Part model, mm, in its own coordinate system. Give positions to 0.01 mm unless a question says otherwise; leave off trailing zeros. Loops run counter-clockwise (first coordinate to the right, second up) from the corner with the lowest first, then second, coordinate; pieces in that order, holes last. Notation, with made-up numbers: (9, 72.5) -> (47, 72.5) arc R11 ccw to (47, 89.5) -> close; hole circle Ø9 at (27.25, 8.25). An arc over 180 degrees is marked (long way). One line per question, with ' | ' between items.
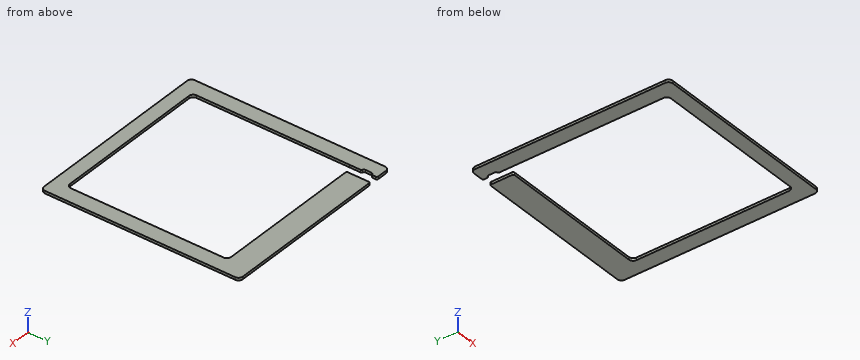
```python
from build123d import *

# Parameters (mm, degrees)
SKETCH1_W           = 323.85
SKETCH1_H           = 336.55
BOSS_EXTRUDE1_DEPTH = 4.3434
SKETCH2_W           = 271.78
SKETCH2_H           = 273.05
CUT_EXTRUDE1_DEPTH  = 5.3434
FILLET1_R           = 7.14375
CUT_EXTRUDE2_DEPTH  = 5.3434
SKETCH4_W           = 14.979655554
SKETCH4_H           = 46.925096095
CUT_EXTRUDE3_DEPTH  = 5.3434
FILLET2_R           = 2.54


with BuildPart() as part:
    # Sketch1 → Boss-Extrude1 (new body)
    with BuildSketch(Plane.XY):
        Rectangle(SKETCH1_W, SKETCH1_H)
    extrude(amount=BOSS_EXTRUDE1_DEPTH)

    # Sketch2 → Cut-Extrude1 (cut, through all)
    with BuildSketch(Plane.XY.offset(4.3434)):
        with Locations((0, -8.382)):
            Rectangle(SKETCH2_W, SKETCH2_H)
    extrude(amount=-CUT_EXTRUDE1_DEPTH, mode=Mode.SUBTRACT)

    # Fillet1
    fillet1_edges = [part.edges().sort_by_distance(p)[0] for p in [
        (135.89, 128.143, 2.1717),
        (135.89, -144.907, 2.1717),
        (-135.89, -144.907, 2.1717),
        (-135.89, 128.143, 2.1717),
        (161.925, -168.275, 2.1717),
        (-161.925, -168.275, 2.1717),
        (-161.925, 168.275, 2.1717),
        (161.925, 168.275, 2.1717),
    ]]
    fillet(fillet1_edges, radius=FILLET1_R)

    # Sketch3 → Cut-Extrude2 (cut, through all)
    with BuildSketch(Plane.XY.offset(4.3434)):
        with BuildLine():
            Line((-139.7, 145.415), (-139.7, 155.575))
            ThreePointArc((-139.7, 155.575), (-136.525, 158.75), (-133.35, 155.575))
            Line((-133.35, 155.575), (-133.35, 145.415))
            ThreePointArc((-133.35, 145.415), (-136.525, 142.24), (-139.7, 145.415))
        make_face()
    extrude(amount=-CUT_EXTRUDE2_DEPTH, mode=Mode.SUBTRACT)

    # Sketch4 → Cut-Extrude3 (cut, through all)
    with BuildSketch(Plane.XY.offset(4.3434)):
        with Locations((-128.400172223, 144.812451952)):
            Rectangle(SKETCH4_W, SKETCH4_H)
    extrude(amount=-CUT_EXTRUDE3_DEPTH, mode=Mode.SUBTRACT)

    # Fillet2
    fillet2_edges = [part.edges().sort_by_distance(p)[0] for p in [
        (-120.910344446, 168.275, 2.1717),
        (-135.89, 142.304148027, 2.1717),
        (-135.89, 168.275, 2.1717),
        (-135.89, 158.685851973, 2.1717),
        (-120.910344446, 128.143, 2.1717),
    ]]
    fillet(fillet2_edges, radius=FILLET2_R)


solid = part.part
```
1) Drill centre lines: line 1 (Y direction, x = 64.5, z = 1.6) (3 decimals); line 2 (X direction, y = -84, z = 2.8) (3 decimals); line 3 (X direction, y = -142, z = 1.4) (3 decimals). Where is each one in solid material? Low to high.
Found:
line 1: -168.275 to -144.907, 128.143 to 168.275 | line 2: -161.925 to -135.89, 135.89 to 161.925 | line 3: -161.925 to -134.498, 134.498 to 161.925
2) Saw through at A-A (y = -35). Give the cut face in (x, z) (3 decimals).
Found:
outline: (-161.925, 0) -> (-135.89, 0) -> (-135.89, 4.343) -> (-161.925, 4.343) -> close; (135.89, 0) -> (161.925, 0) -> (161.925, 4.343) -> (135.89, 4.343) -> close
3) Pin check, flat tip, straight feed: P1, Ø2, axis at y = 163.5, z = 3, coming from the +X side. Stop position of the tip, or through.
Found:
P1: x = 161.79
4) Saw through at B-B (x = 81.5). Give the cut face in (y, z) (3 decimals).
Found:
outline: (-168.275, 0) -> (-144.907, 0) -> (-144.907, 4.343) -> (-168.275, 4.343) -> close; (128.143, 0) -> (168.275, 0) -> (168.275, 4.343) -> (128.143, 4.343) -> close
